Geometry check sheet. Reference: drawing and pictorial views, mm from the part's lowest x, y, z. Round coordinates to 2 decimals unless told otherwise and drop trailing zeros. Order: outer loops, then holes, each group sorted by start corner. A loop starts at its lowest first (then second) coordinate and runs counter-clockwise, first axis right, second up.
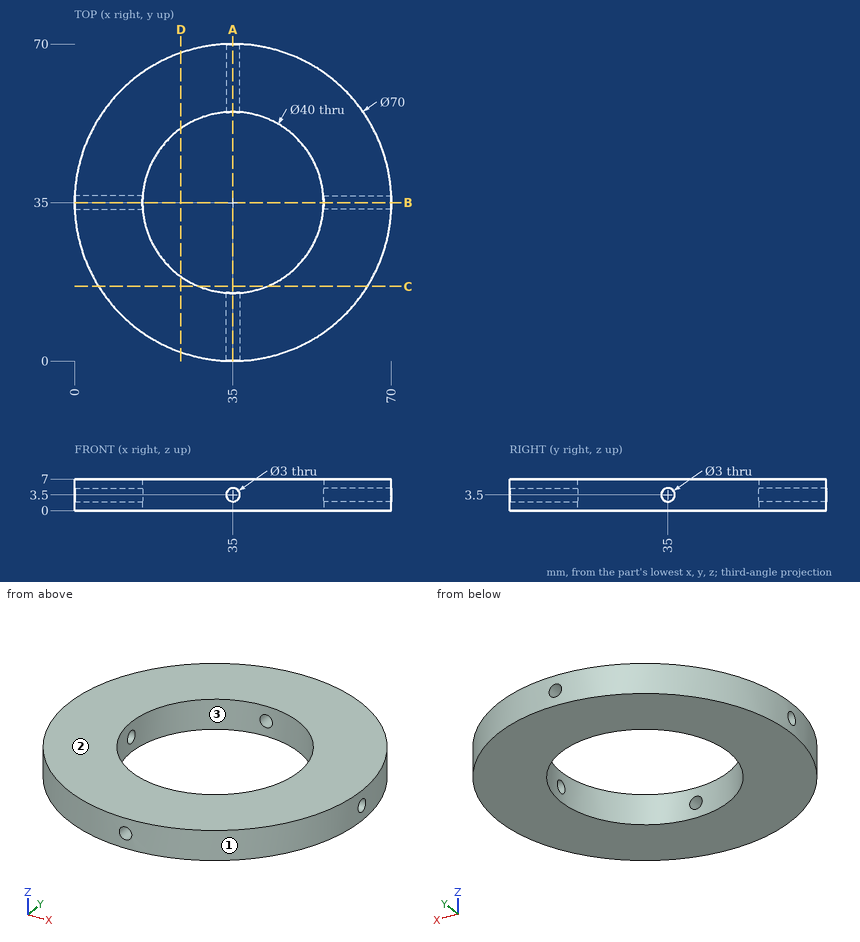
1) Sectioned sample at C-C on y = 16.5. Record the cut outline in (x, z).
2) Go/stop test with flat-tipped pins: pin 1 Ø24 at (x, y) = (35, 35) entering from +Z; pin 2 Ø1.5 at (x, z) = (19, 4) entering from -Y; pin 3 Ø3 at (y, z) = (39, 3) entering from +X. Record where each tip stops, or that it passes through.
3) Sectioned sample at D-D on x = 23.5. Record the cut outline in (y, z).
4) Draft check along Y on the marked faces 1, 2 and 3. Enter one of: released by +Y, released by -Y, zero draft, split by the parting line, or undercut.
5) Scan lines: probe 1 along Z at (x, y) = (35, 63); probe 2 along X at (y, z) = (19.5, 6.5); probe 3 along X at (y, z) = (26, 3.25). Record each from-to range of solid material in increasing order.
6) Sectioned sample at A-A on x = 35. Record the cut outline in (y, z), then the cut area to 3 significant figures.
Returned:
1. outline: (5.29, 0) - (27.4, 0) - (27.4, 7) - (5.29, 7) - close; (42.6, 0) - (64.71, 0) - (64.71, 7) - (42.6, 7) - close
2. pin 1: passes through
2. pin 2: stops at y = 3.5
2. pin 3: stops at x = 69.91
3. outline: (1.94, 0) - (18.64, 0) - (18.64, 7) - (1.94, 7) - close; (51.36, 0) - (68.06, 0) - (68.06, 7) - (51.36, 7) - close
4. face 1: split by the parting line
4. face 2: zero draft
4. face 3: undercut
5. probe 1: z = 0 to 2, 5 to 7
5. probe 2: x = 3.62 to 22.36, 47.64 to 66.38
5. probe 3: x = 1.18 to 17.14, 52.86 to 68.82
6. outline: (0, 0) - (15, 0) - (15, 2) - (0, 2) - close; (0, 5) - (15, 5) - (15, 7) - (0, 7) - close; (55, 0) - (70, 0) - (70, 2) - (55, 2) - close; (55, 5) - (70, 5) - (70, 7) - (55, 7) - close
6. area: 120 mm2
